Verification items for the finished model (mm, model axes). Face numbers are marked on the shaded views. A direction names the side the tool comes from. Round coordinates to 2 decimals unless told otherwise and drop trailing zeros. Order: outer loops, then holes, each group sorted by start corner. A loop starts at its lowest first (then second) coordinate and runs counter-clockwise, first axis right, second up. Notation, with made-up numbers: (68, -24.75) -> (73, -24.75) arc R36 ccw to (73, 10.25) -> close; hole circle Ø4 at (-1.5, 57). An arc over 180 degrees is marked (long way). Put each result on its own line as item: value.
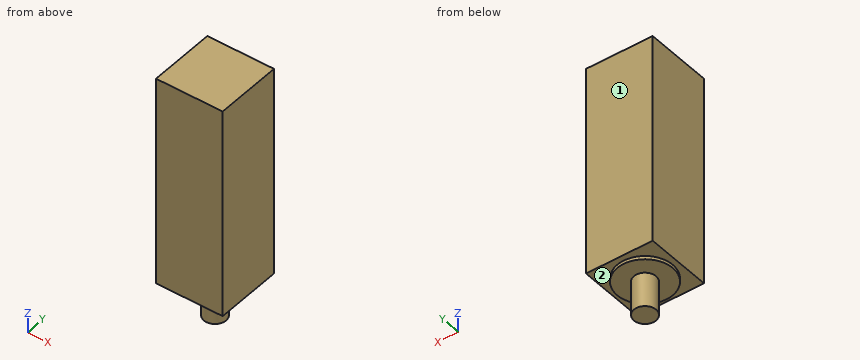
```python
from build123d import *

# Parameters (mm, degrees)
F0_R     = 10
F1_DEPTH = 31
F2_R     = 25
F2_R_2   = 10
F3_DEPTH = 3
F4_W     = 60
F4_H     = 60
F4_R     = 25
F5_DEPTH = 190


with BuildPart() as f1:
    # F0 (on Top) → F1 (new body)
    with BuildSketch(Plane.XY):
        Circle(F0_R)
    extrude(amount=F1_DEPTH)

    # F2 (on face) → F3 (join)
    with BuildSketch(Plane.XY.offset(31)):
        Circle(F2_R)
        Circle(F2_R_2, mode=Mode.SUBTRACT)
        Circle(F2_R_2)
    extrude(amount=F3_DEPTH)

    # F4 (on face) → F5 (join)
    with BuildSketch(Plane.XY.offset(34)):
        Rectangle(F4_W, F4_H)
        Circle(F4_R, mode=Mode.SUBTRACT)
        Circle(F4_R)
    extrude(amount=F5_DEPTH)


solid = f1.part
```
Item 1: Material ranges on line 1 along Z through (x, y) = (17, -12); line 2 along Z through (x, y) = (-13, 24); line 3 along X through (y, z) = (8, 21), recorded low to high.
Geometry check:
line 1: 31 to 224
line 2: 34 to 224
line 3: -6 to 6
Item 2: Sectioned sample at D-D, the plane x = -22.5. Record the boundary of the cut face in (y, z).
Geometry check:
outline: (-30, 34) -> (-10.9, 34) -> (-10.9, 31) -> (10.9, 31) -> (10.9, 34) -> (30, 34) -> (30, 224) -> (-30, 224) -> close
Item 3: Depth check by flat-ended pin: pin 1 Ø1 at (x, y) = (-19, -15.5) entering from -Z. Enter the tip coordinate at first touch or a pass-through.
Geometry check:
pin 1: z = 31
Item 4: Sectioned sample at C-C, the plane y = -20.5. Record the boundary of the cut face in (x, z), then the cut area to 3 significant figures.
Geometry check:
outline: (-30, 34) -> (-14.31, 34) -> (-14.31, 31) -> (14.31, 31) -> (14.31, 34) -> (30, 34) -> (30, 224) -> (-30, 224) -> close
area: 11,500 mm2
Item 5: Sectioned sample at A-A, the plane y = 0. Record the boundary of the cut face in (x, z).
Geometry check:
outline: (-30, 34) -> (-25, 34) -> (-25, 31) -> (-10, 31) -> (-10, 0) -> (10, 0) -> (10, 31) -> (25, 31) -> (25, 34) -> (30, 34) -> (30, 224) -> (-30, 224) -> close
Item 6: Tool access check on the marked faces 1 and 2. Record the directions out of +Z, -Z, +X, -X, +Y, -Y that give a thin tool (end or side, any length) a straight path to the whole face; none if there is none.
Geometry check:
face 1: +Z, -Z, +X, -X, +Y
face 2: -Z
